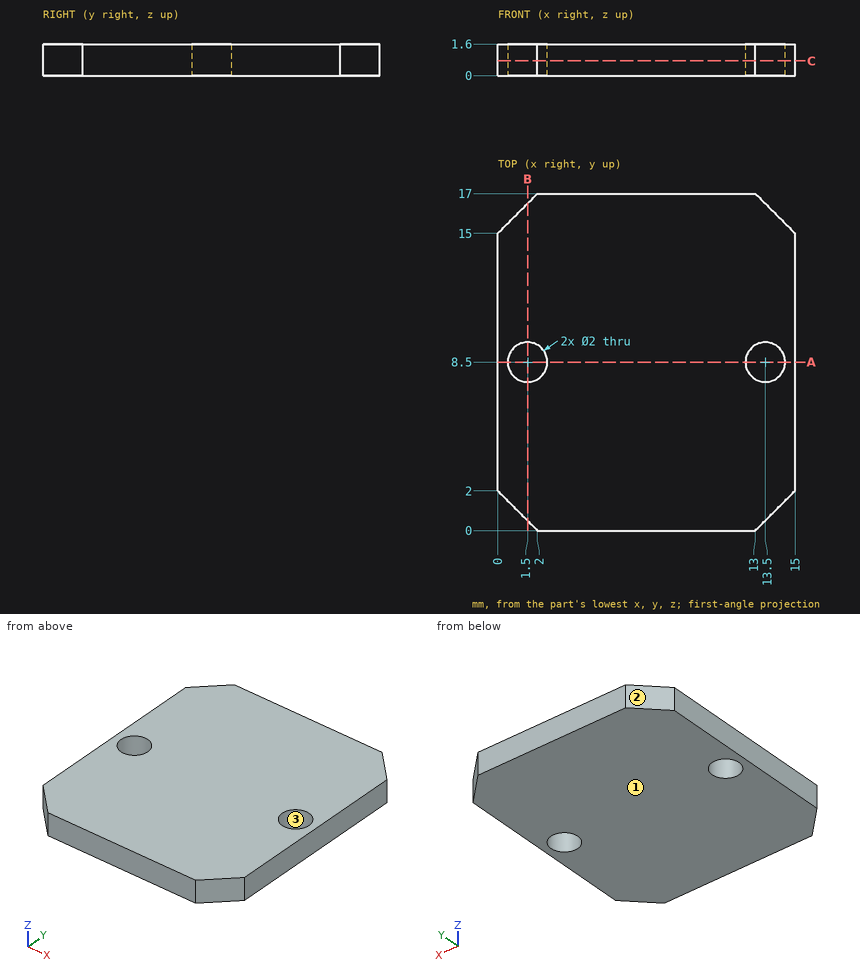
Geometry check sheet. Reference: drawing and pictorial views, mm from the part's lowest x, y, z. Round coordinates to 2 decimals unless told otherwise and drop trailing zeros. Write each loop counter-clockwise with the first axis right and the second up, starting at its lowest first coordinate (ties: lowest second). Pieces come first, ordered by that corner, then holes.
(1) Section check A-A (y = 8.5). Enter the section's corners in (x, z), plus the area to 3 significant figures.
Returned:
outline: (0, 0) - (0.5, 0) - (0.5, 1.6) - (0, 1.6) - close; (2.5, 0) - (12.5, 0) - (12.5, 1.6) - (2.5, 1.6) - close; (14.5, 0) - (15, 0) - (15, 1.6) - (14.5, 1.6) - close
area: 17.6 mm2
(2) Section check B-B (x = 1.5). Enter the section's corners in (y, z).
Returned:
outline: (0.5, 0) - (7.5, 0) - (7.5, 1.6) - (0.5, 1.6) - close; (9.5, 0) - (16.5, 0) - (16.5, 1.6) - (9.5, 1.6) - close
(3) Section check C-C (z = 0.75). Enter the section's corners in (x, y), plus the area to 3 significant figures.
Returned:
outline: (0, 2) - (2, 0) - (13, 0) - (15, 2) - (15, 15) - (13, 17) - (2, 17) - (0, 15) - close; hole circle Ø2 at (1.5, 8.5); hole circle Ø2 at (13.5, 8.5)
area: 241 mm2
(4) Material ranges on line 1 (X direction, y = 8.75, z = 0.5); line 2 (Y direction, x = 1.5, z = 0.3); line 3 (X direction, y = 15.5, z = 1.2), recorded low to high.
Returned:
line 1: x = 0 to 0.53, 2.47 to 12.53, 14.47 to 15
line 2: y = 0.5 to 7.5, 9.5 to 16.5
line 3: x = 0.5 to 14.5
(5) Mould release check, pull along X, two halves, no side actions. Record for the marked faces 1, 2 and 3: pulls with the +X half, pulls with the -X half, needs draft (parallel to the pull), parting line crosses it, or undercut.
Returned:
face 1: needs draft
face 2: pulls with the -X half
face 3: undercut
